Verification items for this drawing (mm, ordinates from the low corner). A direction names the side the tool comes from. Give positions to 0.01 mm unless a question says otherwise; leave off trailing zeros. Loops run counter-clockwise (first coordinate to the right, second up) from the corner with the lowest first, then second, coordinate; pieces in that order, holes last. Notation, with made-up numbers: (4, 64.5) -> (18, 64.5) arc R24 cw to (18, 94.5) -> close; hole circle Ø7 at (-9.5, 56.25). An arc over 180 degrees is marked (long way). Write each question's results on one line, items separated by ' | '. Start each with the question number.
1) Sectioned sample at A-A on y = 25. Record the cut outline in (x, z) (1 decimal).
2) Draft check along X on the marked faces 1, 2 and 3. Enter one of: pulls with the +X half, pulls with the -X half, needs draft (parallel to the pull), parting line crosses it, or undercut.
3) Set-up check for the marked faces 4 and 5: record each of +Z, -Z, +X, -X, +Y, -Y from which the full face is reachable in a straight line by a thin tool's end or side.
4) Scan lines: line 1 (Y direction, x = 25, z = 3.9) (1 decimal); line 2 (Z direction, x = 17.5, y = 16.5); line 3 (Y direction, x = 11.5, z = 15.25) (1 decimal). Record each from-to range of solid material in increasing order. Write a range as from..to.
5) Sectioned sample at B-B on x = 25. Record the cut outline in (y, z) (1 decimal), then the cut area to 3 significant figures.
6) Sectioned sample at D-D on x = 36.5. Record the cut outline in (y, z).
7) Depth check by flat-ended pin: pin 1 (5 mm diameter, centred on y = 30, z = 13, fed in from +X); pin 2 (5 mm diameter, centred on x = 16.5, z = 14, fed in from +Y); pin 3 (1 mm diameter, centred on x = 15, z = 3.5, fed in from +Y) (1 decimal). Enter the tip coordinate at first touch or a pass-through.
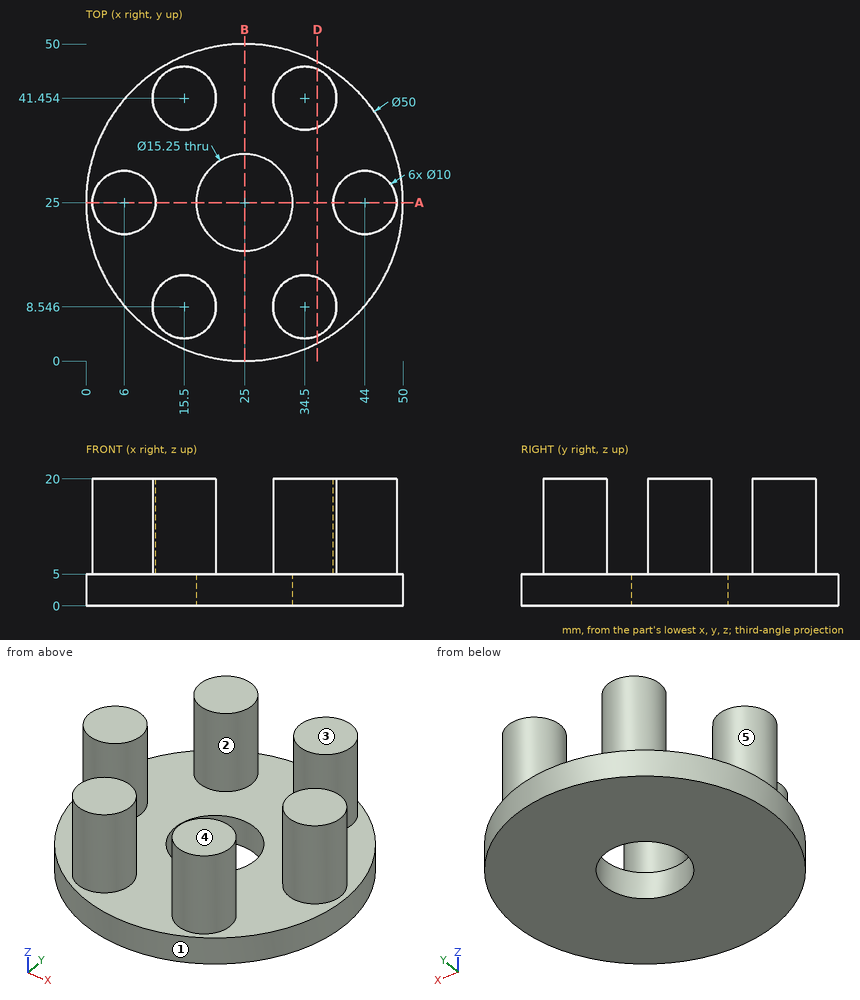
Result:
1) outline: (0, 0) -> (17.4, 0) -> (17.4, 5) -> (11, 5) -> (11, 20) -> (1, 20) -> (1, 5) -> (0, 5) -> close; (32.6, 0) -> (50, 0) -> (50, 5) -> (49, 5) -> (49, 20) -> (39, 20) -> (39, 5) -> (32.6, 5) -> close
2) face 1: parting line crosses it | face 2: undercut | face 3: needs draft
3) face 4: +Z, +X, -X, +Y, -Y | face 5: +Z
4) line 1: 0..17.4, 32.6..50 | line 2: 0..5 | line 3: 5.5..11.5, 38.5..44.5
5) outline: (0, 0) -> (17.4, 0) -> (17.4, 5) -> (0, 5) -> close; (32.6, 0) -> (50, 0) -> (50, 5) -> (32.6, 5) -> close | area: 174 mm^2
6) outline: (2.8, 0) -> (47.2, 0) -> (47.2, 5) -> (46.04, 5) -> (46.04, 20) -> (36.87, 20) -> (36.87, 5) -> (13.13, 5) -> (13.13, 20) -> (3.96, 20) -> (3.96, 5) -> (2.8, 5) -> close
7) pin 1: x = 48.33 | pin 2: y = 46.45 | pin 3: y = 48.1
